```python
from build123d import *

# Parameters (mm, degrees)
SKETCH1_R        = 2.5
BASENUT_DEPTH    = 5
ENDCHAMFER_SIZE  = 0.65
ENDCHAMFER_SIZE2 = 0.375277675


with BuildPart() as part:
    # Sketch1 → BaseNut (new body)
    with BuildSketch(Plane.XY):
        Polygon((5.646485633, 0), (2.823242816, 4.89), (-2.823242816, 4.89), (-5.646485633, 0), (-2.823242816, -4.89), (2.823242816, -4.89), align=None)
        Circle(SKETCH1_R, mode=Mode.SUBTRACT)
    extrude(amount=-BASENUT_DEPTH)

    # Sketch2 → DoubleChamfer (revolve, cut)
    with BuildSketch(Plane(origin=(0, 0, 0), x_dir=(1, 0, 0), z_dir=(0, 1, 0))):
        Polygon((-4.89, 5), (-5.646485633, 5), (-5.646485633, 4.724661747), align=None)
        Polygon((-5.646485633, 0.275338253), (-4.89, 0), (-5.646485633, 0), align=None)
    revolve(axis=Axis((0, 0, -3.377940403), (0, 0, 1)), mode=Mode.SUBTRACT)

    # Sketch3 → Crown (revolve)
    with BuildSketch(Plane(origin=(-4.6, 0, -6), x_dir=(-1, 0, 0), z_dir=(0, 1, 0))):
        with BuildLine():
            Line((-9.2, 7.4), (-9.2, 6))
            Line((-9.2, 6), (-7.85, 6))
            Line((-7.85, 6), (-7.85, 8))
            Line((-7.85, 8), (-4.6, 11))
            Line((-4.6, 11), (-4.6, 12))
            ThreePointArc((-4.6, 12), (-7.852691193, 10.652691193), (-9.2, 7.4))
        make_face()
    revolve(axis=Axis((0, 0, 6), (0, 0, -1)))

    # EndChamfer
    endchamfer_edges = [part.edges().sort_by_distance(p)[0] for p in [
        (-2.5, 0, -5),
    ]]
    endchamfer_side = [part.faces().sort_by_distance(p)[0] for p in [
        (-2.5, 0, -2.5),
    ]]
    chamfer(endchamfer_edges, length=ENDCHAMFER_SIZE, length2=ENDCHAMFER_SIZE2, reference=endchamfer_side[0])


solid = part.part
```
Check sheet for the modelled part. Datum: model origin and axes. Units: mm. A direction names the side the tool comes from. Give positions to 0.01 mm unless a question says otherwise; leave off trailing zeros. Loops run counter-clockwise (first coordinate to the right, second up) from the corner with the lowest first, then second, coordinate; pieces in that order, holes last. Notation, with made-up numbers: M 75.25,32.5 L 117.25,32.5 A4 cw 117.25,36.5 Z; hole C -9.5,1 d10. An arc over 180 degrees is marked long. Answer as CSV lines item,"result".
Item 1: Scan lines: L1, parallel to Y at x = 0, z = 1.2; L2, parallel to Y at x = 0.5, z = -1.25. Record each from-to range of solid material in increasing order.
Reply:
L1,"-4.6 to -3.25, 3.25 to 4.6"
L2,"-4.89 to -2.45, 2.45 to 4.89"
Item 2: Sectioned sample at A-A, the plane z = -2.25. Enter the section's corners in (x, y), then the cut area to 3 significant figures.
Reply:
outline,"M -5.65,0 L -2.82,-4.89 L 2.82,-4.89 L 5.65,0 L 2.82,4.89 L -2.82,4.89 Z; hole C 0,0 d5"
area,"63.2 mm^2"
Item 3: Sectioned sample at D-D, the plane z = 2.75. Enter the section's corners in (x, y) (1 decimal), then the cut area to 3 significant figures.
Reply:
outline,"C 0,0 d8.8; hole C 0,0 d4.9"
area,"42.1 mm^2"
Item 4: Draft check along Y on faces 1 (the face through (5.07, -0.012, -4.934)), 2 (the face through (-0.54, -2.44, -2.14)), 3 (the face through (4.255, 2.411, -2.465)). Enter one of: pulls with the +Y half, pulls with the -Y half, needs draft (parallel to the pull), parting line crosses it, or undercut.
Reply:
face 1,"parting line crosses it"
face 2,"undercut"
face 3,"pulls with the +Y half"
Item 5: Set-up check for faces 4 (the face through (-3.65, 2.8, 0.69)), 5 (the face through (0.84, -0.26, 4.19)), 6 (the face through (5.07, -0.012, -0.066)): record each of +Z, -Z, +X, -X, +Y, -Y from which the full face is reachable in a straight line by a thin tool's end or side.
Reply:
face 4,"+Z"
face 5,"none"
face 6,"+Z, +X"
Item 6: Sectioned sample at C-C, the plane z = 5.25. Enter the section's corners in (x, y).
Reply:
outline,"C 0,0 d5.03"
Item 7: Depth check by flat-ended pin: pin 1 Ø2 at (y, z) = (3, -2.5) entering from +X; pin 2 Ø1.5 at (y, z) = (2, 3) entering from +X; pin 3 Ø3 at (x, z) = (4.5, 2) entering from -Y. Enter the tip coordinate at first touch or a pass-through.
Reply:
pin 1,"x = 4.49"
pin 2,"x = 4.23"
pin 3,"y = -3.45"
Item 8: Sectioned sample at B-B, the plane z = 1. Enter the section's corners in (x, y), then the cut area to 3 significant figures.
Reply:
outline,"C 0,0 d9.2; hole C 0,0 d6.5"
area,"33.3 mm^2"
